Could you check a few things on this model? Use its own coordinates, in mm. Face numbers are marked on the shaded views. A direction names the side the tool comes from. Round coordinates to 2 decimals unless told otherwise and drop trailing zeros. Loops run counter-clockwise (first coordinate to the right, second up) from the corner with the lowest first, then second, coordinate; pieces in that order, holes last. Notation, with made-up numbers: (58, -36.5) -> (63, -36.5) arc R15 ccw to (63, -22.5) -> close; hole circle Ø6 at (39.25, 63.25). An arc over 180 degrees is marked (long way). Write each question's results on one line, items separated by ' | '.
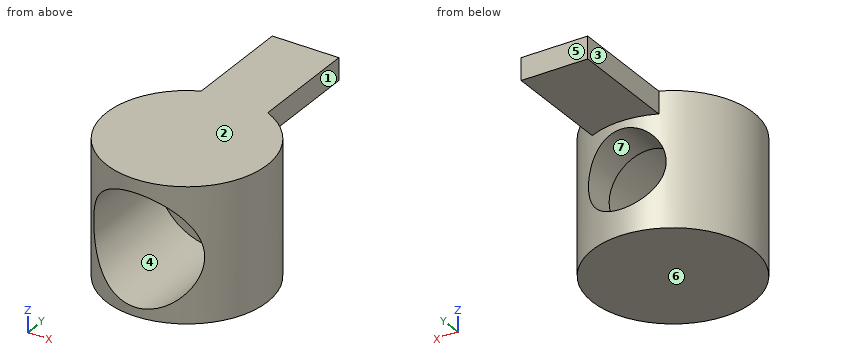
from build123d import *

# Parameters (mm, degrees)
SKETCH_1_W               = 6
SKETCH_1_H               = 23
EXTRUDE_1_DEPTH          = 2
SKETCH_4_W               = 6
SKETCH_4_H               = 4.448435562
CUT_EXTRUDE_1_DEPTH      = 13.051970793
SKETCH_2_R               = 7.25
EXTRUDE_2_DEPTH          = 12
SKETCH_5_R               = 3.5
CUT_EXTRUDE_2_DEPTH      = 27.752110197
CUT_EXTRUDE_3_DEPTH      = 2.75
CUT_EXTRUDE_3_DEPTH_BACK = 10
SKETCH_6_R               = 5


with BuildPart() as part:
    # 草图1 → 凸台-拉伸1 (new body)
    with BuildSketch(Plane.XY):
        Rectangle(SKETCH_1_W, SKETCH_1_H)
    extrude(amount=EXTRUDE_1_DEPTH)

    # 草图4 → 切除-拉伸1 (cut, through all)
    with BuildSketch(Plane(origin=(0, 0, 0), x_dir=(-1, 0, 0), z_dir=(0, 0, -1))):
        with Locations((0, -9.275782219)):
            Rectangle(SKETCH_4_W, SKETCH_4_H)
    extrude(amount=-CUT_EXTRUDE_1_DEPTH, mode=Mode.SUBTRACT)

    # 草图2 → 凸台-拉伸2 (add)
    with BuildSketch(Plane.XY.offset(2)):
        with Locations((0, -4.98)):
            Circle(SKETCH_2_R)
    extrude(amount=-EXTRUDE_2_DEPTH)

    # 草图5 → 切除-拉伸2 (cut, through all)
    with BuildSketch(Plane(origin=(0, 11.5, 0), x_dir=(1, 0, 0), z_dir=(0, 1, 0))):
        with Locations(Location((0, 4.2, 0), (0, 0, 270))):
            Circle(SKETCH_5_R)
    extrude(amount=-CUT_EXTRUDE_2_DEPTH, mode=Mode.SUBTRACT)

    # 草图6 → 切除-拉伸3 (cut, two sides: drawn at the far end of the back side and taken through both)
    with BuildSketch(Plane(origin=(0, -4.25, 0), x_dir=(1, 0, 0), z_dir=(0, 1, 0)).offset(-CUT_EXTRUDE_3_DEPTH_BACK)):
        with Locations(Location((0, 4.2, 0), (0, 0, 90))):
            Circle(SKETCH_6_R)
    extrude(amount=CUT_EXTRUDE_3_DEPTH + CUT_EXTRUDE_3_DEPTH_BACK, mode=Mode.SUBTRACT)


solid = part.part
1) I need wall thicknesses on line 1 (Z direction, x = 0, y = 1.1); line 2 (X direction, y = -3.75, z = -2.5); line 3 (X direction, y = -7.25, z = -4.2). Which ranges of each line are inside material? Lowest first, please.
Model answer:
line 1: z = -10 to -7.7, -0.7 to 2 | line 2: x = -7.14 to -4.7, 4.7 to 7.14 | line 3: x = -6.89 to -5, 5 to 6.89
2) I want a section at D-D, the plane z = -2. Write out the boundary of the cut face in (x, y), plus the area to 3 significant figures.
Model answer:
outline: (-4.49, -10.67) -> (-4.49, -1.5) -> (-2.72, -1.5) -> (-2.72, 1.74) arc R7.25 ccw to start; (2.72, -1.5) -> (4.49, -1.5) -> (4.49, -10.67) arc R7.25 ccw to (2.72, 1.74) -> close | area: 53.6 mm2
3) I want a section at C-C, the plane y = -4.98. Write out the boundary of the cut face in (x, z).
Model answer:
outline: (-7.25, -10) -> (7.25, -10) -> (7.25, 2) -> (-7.25, 2) -> close; hole circle Ø10 at (0, -4.2)
4) I'm going to push flat-ended pins straight in: pin 1 (2 mm diameter, centred on y = 7.5, z = 1, fed in from +X); pin 2 (1 mm diameter, centred on y = 1.5, z = -7, fed in from -X); pin 3 (3 mm diameter, centred on x = 3.5, y = 8.5, fed in from -Z). Where does each tip first touch, or does it pass through?
Model answer:
pin 1: stops at x = 3 | pin 2: stops at x = -4.1 | pin 3: stops at z = 0
5) For the marked faces 1, 2, 3 and 4, which set-ups out of +Z, -Z, +X, -X, +Y, -Y let a thin tool reach every point of the face, with its end or its side?
Model answer:
face 1: +Z, -Z, +X, +Y | face 2: +Z, +X, -X, +Y, -Y | face 3: +Z, -Z, -X, +Y | face 4: -Y
6) I want a section at A-A, the plane x = 0. Write out the boundary of the cut face in (y, z).
Model answer:
outline: (-12.23, -10) -> (2.27, -10) -> (2.27, -7.7) -> (-1.5, -7.7) -> (-1.5, -9.2) -> (-12.23, -9.2) -> close; (-12.23, 0.8) -> (-1.5, 0.8) -> (-1.5, -0.7) -> (2.27, -0.7) -> (2.27, 0) -> (11.5, 0) -> (11.5, 2) -> (-12.23, 2) -> close
7) If we mould it in two halves opening along Z, with no side actions, what happens to the marked faces 5, 6 and 7? For each: released by +Z, released by -Z, zero draft, split by the parting line, or undercut.
Model answer:
face 5: zero draft | face 6: released by -Z | face 7: undercut
8) I want a section at B-B, the plane z = -4.2. Write out the boundary of the cut face in (x, y), plus the area to 3 significant figures.
Model answer:
outline: (-5, -10.23) -> (-5, -1.5) -> (-3.5, -1.5) -> (-3.5, 1.37) arc R7.25 ccw to start; (3.5, -1.5) -> (5, -1.5) -> (5, -10.23) arc R7.25 ccw to (3.5, 1.37) -> close | area: 39.7 mm2
